Source: three-view drawing plus pictorial views. Frame: mm from the lowest corner of the part. Round coordinates to 2 decimals unless told otherwise and drop trailing zeros. Order: outer loops, then holes, each group sorted by start corner. A loop starts at its lowest first (then second) coordinate and runs counter-clockwise, first axis right, second up. Notation, with made-up numbers: (20.5, 29) -> (33.5, 29) arc R23 ccw to (33.5, 55) -> close; hole circle Ø2 at (2, 25). An arc over 180 degrees is marked (long way). Use a Markdown table: item, result.
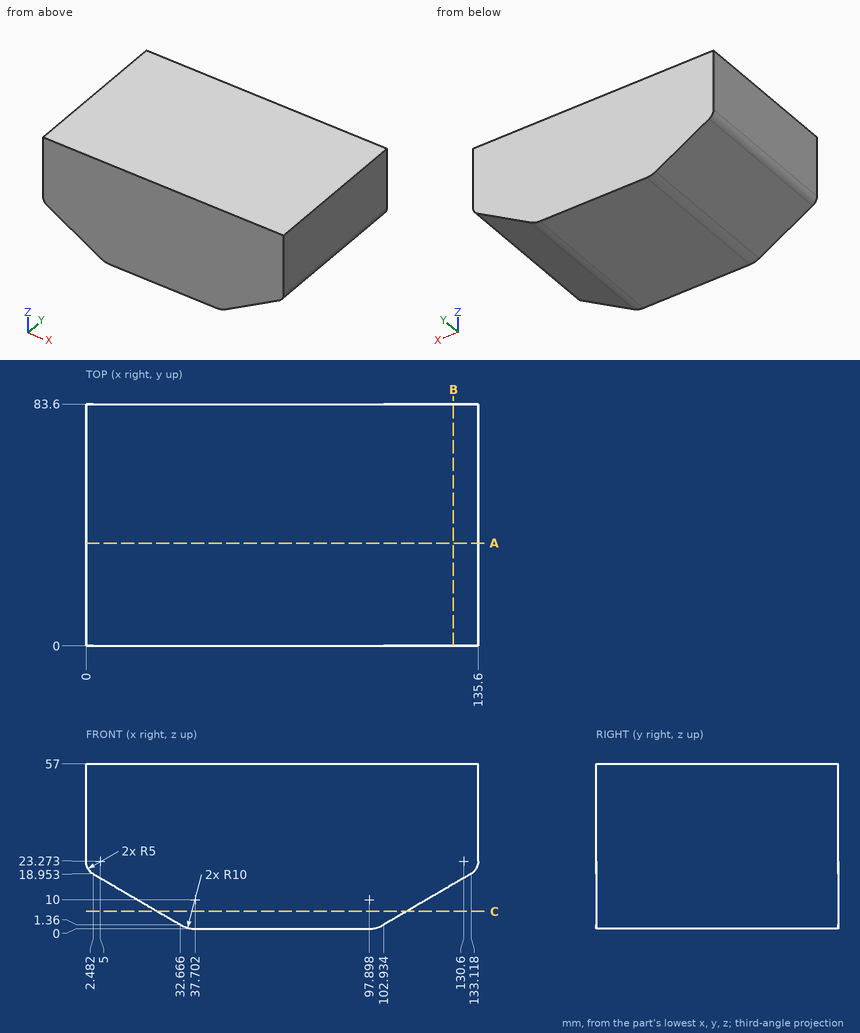
1) Cut plane A-A on y = 35.5. Return loops of the section in (x, z).
Results found:
| item | result |
|---|---|
| outline | (0, 23.27) arc R5 ccw to (2.48, 18.95) -> (32.67, 1.36) arc R10 ccw to (37.7, 0) -> (97.9, 0) arc R10 ccw to (102.93, 1.36) -> (133.12, 18.95) arc R5 ccw to (135.6, 23.27) -> (135.6, 57) -> (0, 57) -> close |
2) Pin query (flat end, axial travel): pin 1 Ø3 at (y, z) = (63.5, 15) entering from -X; pin 2 Ø5 at (x, y) = (32.5, 23) entering from -Z; pin 3 Ø2 at (x, y) = (111, 44) entering from -Z. Return the tip coordinate at first contact, or that it passes through.
Results found:
| item | result |
|---|---|
| pin 1 | stops at x = 6.69 |
| pin 2 | stops at z = 0.37 |
| pin 3 | stops at z = 5.48 |
3) Cut plane C-C on z = 6. Return loops of the section in (x, y).
Results found:
| item | result |
|---|---|
| outline | (24.71, 0) -> (110.89, 0) -> (110.89, 83.6) -> (24.71, 83.6) -> close |
4) Cut plane B-B on x = 127. Return loops of the section in (y, z), and give its area (3 significant figures).
Results found:
| item | result |
|---|---|
| outline | (0, 15.39) -> (83.6, 15.39) -> (83.6, 57) -> (0, 57) -> close |
| area | 3,480 mm² |
5) Line query: L1, parallel to X at y = 4.5, z = 23; L2, parallel to X at y = 24.5, z = 5 (1 decimal); L3, parallel to Z at x = 104.5, y = 72. Output: solid intervals per line, ascending. Write a range as [from, to].
Results found:
| item | result |
|---|---|
| L1 | x = [0.01, 135.59] |
| L2 | x = [26.4, 109.2] |
| L3 | z = [2.27, 57] |
